from build123d import *

# Parameters (mm, degrees)
SKETCH7_R                = 4
SKETCH7_R_2              = 2
BOSS_EXTRUDE1_DEPTH      = 5
HOLE_WIZARD_M3_5_1_D     = 3.9
HOLE_WIZARD_M3_5_1_DEPTH = 10
HOLE_WIZARD_M3_5_1_TIP   = 1.171678207
SKETCH_4_R               = 1.75
CUT_EXTRUDE_1_DEPTH      = 10


with BuildPart() as part:
    # Sketch7 → Boss-Extrude1 (new body)
    with BuildSketch(Plane.XY):
        with BuildLine():
            Line((8.994200014, 237.123057432), (17.48872225, 0.62816723))
            ThreePointArc((17.48872225, 0.62816723), (0, -17.5), (-17.48872225, 0.62816723))
            Line((-17.48872225, 0.62816723), (-8.994200014, 237.123057432))
            ThreePointArc((-8.994200014, 237.123057432), (0, 245.8), (8.994200014, 237.123057432))
        make_face()
        Circle(SKETCH7_R, mode=Mode.SUBTRACT)
        with Locations((0, 236.8)):
            Circle(SKETCH7_R_2, mode=Mode.SUBTRACT)
    extrude(amount=-BOSS_EXTRUDE1_DEPTH)

    # M3.5 间隙孔1
    with Locations(Plane(origin=(0, 156.8, 0), x_dir=(1, 0, 0), z_dir=(0, 0, 1))):
        with Locations((0, 0), (0, -76.8)):
            Hole(HOLE_WIZARD_M3_5_1_D / 2, depth=HOLE_WIZARD_M3_5_1_DEPTH)
            with Locations((0, 0, -(HOLE_WIZARD_M3_5_1_DEPTH + HOLE_WIZARD_M3_5_1_TIP / 2))):  # 118° drill point
                Cone(0, HOLE_WIZARD_M3_5_1_D / 2, HOLE_WIZARD_M3_5_1_TIP, mode=Mode.SUBTRACT)

    # 草图4 → 切除-拉伸1 (cut)
    with BuildSketch(Plane.XY):
        with Locations((7, 0)):
            Circle(SKETCH_4_R)
        with Locations((0, 7)):
            Circle(SKETCH_4_R)
        with Locations((0, -7)):
            Circle(SKETCH_4_R)
        with Locations((-7, 0)):
            Circle(SKETCH_4_R)
    extrude(amount=-CUT_EXTRUDE_1_DEPTH, mode=Mode.SUBTRACT)


solid = part.part
Read the model definition and answer for the solid it produces. Units are mm, in the model's axes. Round coordinates to 2 decimals unless told otherwise and drop trailing zeros. Order: outer loops, then holes, each group sorted by start corner. A loop starts at its lowest first (then second) coordinate and runs counter-clockwise, first axis right, second up.
1) A flat-ended cylindrical pin translates along its axis: pin 1 (6.5 mm diameter, centred on x = 0, y = 0, fed in from +Z). Find the tip coordinate at first contact, or state that the pin passes through.
2) The part is cut by section C-C on x = -12.5. Write down the section's boundary in (y, z).
3) The mould has two halves that part along Y. Classify faces 1 (the face through (-0.867, -3.905, -2.465)), 2 (the face through (0, 116, -5)), 3 (the face through (-0.193, 245.798, -2.465)): released by +Y, released by -Y, zero draft, split by the parting line, or undercut.
4) Straight lines are drawn through the part: L1, parallel to Y at x = 3, z = -3.5; L2, parallel to Y at x = -7, z = -3; L3, parallel to X at y = 214.5, z = -3.1. For each, find the intervals that lie inside material, in ascending order.
5) The part is cut by section A-A on z = -2.3. Give the number of separate pieces and of enclosed holes in the cut face, plus the area to 3 significant figures.
6) The part is cut by section B-B on y = 185.5. Write down the section's boundary in (x, z), plus the area to 3 significant figures.
Resolved:
1. pin 1: passes through
2. outline: (-12.25, -5) - (139.52, -5) - (139.52, 0) - (-12.25, 0) - close
3. face 1: undercut
3. face 2: zero draft
3. face 3: released by +Y
4. L1: y = -17.24 to -2.65, 2.65 to 245.29
4. L2: y = -16.04 to -1.75, 1.75 to 242.46
4. L3: x = -9.81 to 9.81
5. separate pieces: 1
5. enclosed holes: 8
5. area: 6,760 mm2
6. outline: (-10.85, -5) - (10.85, -5) - (10.85, 0) - (-10.85, 0) - close
6. area: 108 mm2
